Check sheet for the modelled part. Datum: model origin and axes. Units: mm. A direction names the side the tool comes from. Round coordinates to 2 decimals unless told otherwise and drop trailing zeros. Write each loop counter-clockwise with the first axis right and the second up, starting at its lowest first coordinate (ties: lowest second). Pieces come first, ordered by that corner, then holes.
Item 1: Cross-section at A-A on y = 10.25. Enter the section's corners in (x, z), plus the area to 3 significant figures.
Item 2: Tool access check on faces 1 (the flat face through (10, 25, 18)), 2 (the flat face through (5.024, 24.236, 0.304)), 3 (the flat face through (14.956, 24.162, 0.304)). Record the directions out of +Z, -Z, +X, -X, +Y, -Y that give a thin tool (end or side, any length) a straight path to the whole face; none if there is none.
Item 3: Go/stop test with a flat-tipped pin: pin 1 Ø3.5 at (x, y) = (10, 25) entering from +Z. Record where the tip stops, or that it passes through.
Item 4: Release check for a two-part mould opening along Y. For faces 4 (the flat face through (15.344, 24.468, 9.178)), 5 (the flat face through (10, 26.75, 9)), 6 (the flat face through (20, 11, 10)), 7 (the flat face through (10, 0, 10)) record: +Y half, -Y half, draft (parallel to the pull), parting line (faces both ways), or undercut.
Item 5: Material ranges on line 1 (Y direction, x = 10, z = 15.25); line 2 (X direction, y = 10, z = 15.75); line 3 (Z direction, x = 7.75, y = 24), recorded low to high.
Item 6: Cross-section at C-C on x = 10. Enter the section's corners in (y, z).
Item 7: Cross-section at B-B on z = 9.75. Enter the section's corners in (x, y).
Item 8: Cross-section at D-D on x = 18.25. Enter the section's corners in (y, z), plus the area to 3 significant figures.
from build123d import *

# Parameters (mm, degrees)
F2_R     = 5.25
F3_DEPTH = 20
F4_DEPTH = 18
F5_SIZE  = 0.6


# Not quite as in the source:
# - a feature names something its author has since deleted; it is built from what else it names


with BuildPart() as f3:
    # F2 (on Top) → F3 (new body)
    with BuildSketch(Plane.XY):
        Polygon((5.25, 22.25), (0, 22.25), (0, 0), (20, 0), (20, 22.25), (14.75, 22.25), align=None)
        with Locations((10, 10.25)):
            Circle(F2_R, mode=Mode.SUBTRACT)
    extrude(amount=F3_DEPTH)

    # F2 (on Top) → F4 (join)
    with BuildSketch(Plane.XY):
        Polygon((4.0442286341, 26.75), (5.25, 22.25), (14.75, 22.25), (15.9557713659, 26.75), align=None)
    extrude(amount=F4_DEPTH)

    # F5
    f5_edges = [f3.edges().sort_by_distance(p)[0] for p in [
        (0, 11.125, 0),
        (10, 0, 0),
        (20, 11.125, 0),
        (17.375, 22.25, 0),
        (15.352886, 24.5, 0),
        (10, 26.75, 0),
        (4.647114, 24.5, 0),
        (2.625, 22.25, 0),
        (4.75, 10.25, 0),
        (10, 22.25, 20),
        (0, 11.125, 20),
        (10, 0, 20),
        (20, 11.125, 20),
        (4.75, 10.25, 20),
        (0, 0, 10),
        (20, 0, 10),
        (20, 22.25, 10),
    ]]
    chamfer(f5_edges, length=F5_SIZE)


solid = f3.part
Response values:
1. outline: (0, 0.6) - (0.6, 0) - (4.15, 0) - (4.75, 0.6) - (4.75, 19.4) - (4.15, 20) - (0.6, 20) - (0, 19.4) - close; (15.25, 0.6) - (15.85, 0) - (19.4, 0) - (20, 0.6) - (20, 19.4) - (19.4, 20) - (15.85, 20) - (15.25, 19.4) - close
1. area: 189 mm2
2. face 1: +Z, +X, -X, +Y
2. face 2: -Z, -X
2. face 3: -Z, +X
3. pin 1: stops at z = 18
4. face 4: undercut
4. face 5: +Y half
4. face 6: draft
4. face 7: -Y half
5. line 1: y = 0 to 5, 15.5 to 26.75
5. line 2: x = 0 to 4.76, 15.24 to 20
5. line 3: z = 0 to 18
6. outline: (0, 0.6) - (0.6, 0) - (4.4, 0) - (5, 0.6) - (5, 19.4) - (4.4, 20) - (0.6, 20) - (0, 19.4) - close; (15.5, 0.6) - (16.1, 0) - (26.15, 0) - (26.75, 0.6) - (26.75, 18) - (22.25, 18) - (22.25, 19.4) - (21.65, 20) - (16.1, 20) - (15.5, 19.4) - close
7. outline: (0, 0.6) - (0.6, 0) - (19.4, 0) - (20, 0.6) - (20, 21.65) - (19.4, 22.25) - (14.75, 22.25) - (15.96, 26.75) - (4.04, 26.75) - (5.25, 22.25) - (0, 22.25) - close; hole circle Ø10.5 at (10, 10.25)
8. outline: (0, 0.6) - (0.6, 0) - (21.65, 0) - (22.25, 0.6) - (22.25, 19.4) - (21.65, 20) - (0.6, 20) - (0, 19.4) - close
8. area: 444 mm2
